Source: CAD feature listing. Evaluate the final solid. Frame: model axes, mm. A direction names the side the tool comes from. Coordinates: 2 decimals unless noted, no trailing zeros. Write each loop counter-clockwise with the first axis right and the second up, starting at its lowest first coordinate (ties: lowest second). Pieces come first, ordered by that corner, then holes. Notation, with made-up numbers: M 87.5,63.25 L 133.5,63.25 A28 cw 133.5,85.25 Z; hole C 10.5,-33 d5. An arc over 180 degrees is marked long. Answer as CSV lines item,"result". Start each with the question number.
1. Line query: probe 1 along Y at (x, z) = (-7.5, 484.05); probe 2 along Z at (x, y) = (-7.5, -4.25); probe 3 along Z at (x, y) = (7.5, -6.25). Output: solid intervals per line, ascending. Write a range as [from, to].
2. Contact query for flat-ended pins moving along their axis: pin 1 Ø1 at (x, z) = (0.5, 265.5) entering from +Y; pin 2 Ø1.5 at (x, z) = (-2, 96) entering from +Y; pin 3 Ø1.5 at (x, y) = (-4.5, -15) entering from +Z; pin 4 Ø0.6 at (x, z) = (1, 337.5) entering from -Y. Output: stop coordinate, or through.
3. Reachability of faces 4 (the face through (-7, -16, 0)), 5 (the face through (18.53, -8.73, 494.61)), 6 (the face through (16.5, -13.8, 480)) from +Z, -Z, +X, -X, +Y, -Y: full face, straight path, thin tool, end or side. Return the list, or none.
4. Mould query, pull axis Z, two halves, no side actions, for faces 1 (the face through (16, -15, 505)), 2 (the face through (0, -14, 243)), 3 (the face through (14, 0, 243)). Classes: pulls with the +Z half, pulls with the -Z half, needs draft (parallel to the pull), parting line crosses it, or undercut.
5. Section A-A on z = 353. Return the cut outline in (x, y), plus the area to 3 significant figures.
Autodesk Inventor part; units mm, degrees
ref_plane "YZ Plane" through (0, 0, 0) normal (1, 0, 0) x (0, 1, 0)
ref_plane "XZ Plane" through (0, 0, 0) normal (0, 1, 0) x (-1, 0, 0)
ref_plane "XY Plane" through (0, 0, 0) normal (0, 0, 1) x (1, 0, 0)
sketch "草图1" plane through (0, 0, 0) normal (0, 0, 1) x (1, 0, 0)
  arc A0 (0, -28) -> (28, 0) centre (0, 0) ccw
  line L0 (0, 0) -> (28, 0)
  line L1 (0, 0) -> (0, -28)
  dimension "d0" = 28
extrude "拉伸1" add sketch "草图1" along normal blind 480
shell "抽壳1" thickness 2 removed faces 1 at (13.1163, -13.1163, 480)
sketch "草图2" plane through (0, 0, 480) normal (0, 0, 1) x (1, 0, 0)
  line L0 (0, -28) -> (-15, -28)
  line L1 (-15, -28) -> (-15, 0)
  line L2 (-15, 0) -> (0, 0)
  line L3 (0, 0) -> (0, -28)
  line L4 (28, 0) -> (0, 0)
  arc A0 (0, -28) -> (28, 0) centre (0, 0) ccw
  line L5 (0, 0) -> (28, 0)
  line L6 (0, 0) -> (0, -28)
  line L7 (0, 0) -> (0, -28)
  dimension "d4" = 15
extrude "拉伸2" add sketch "草图2" along normal blind 5
sketch "草图3" plane through (0, 0, 485) normal (0, 0, 1) x (1, 0, 0)
  circle A0 centre (11.598, -11.598) radius 7.5
  circle A1 centre (11.598, -11.598) radius 11.598
  line L0 (28, 0) -> (-15, 0)
  line L1 (0, 0) -> (0, -28)
  arc A2 (0, -28) -> (28, 0) centre (0, 0) ccw
  dimension "d7" = 15
extrude "拉伸3" add sketch "草图3" along normal blind 20 contours A0
sketch "草图4" plane through (11.598, -11.598, 505) normal (0, 0, 1) x (1, 0, 0)
  circle A0 centre (0, 0) radius 5
  circle A1 centre (0, 0) radius 7.5
  point P0 (-11.598, 11.598)
  dimension "d10" = 10
extrude "拉伸4" cut sketch "草图4" against normal up to surface (25 mm away) contours A0
thread "螺纹1"
chamfer "倒角1" distance 0.5 angle 45 1 edges at (4.098, -11.598, 505)
sketch "草图5" plane through (0, 0, 0) normal (0, 0, -1) x (-1, 0, 0)
  arc A0 (-28, 0) -> (0, -28) centre (0, 0) ccw
  line L0 (-28, 0) -> (15, 0)
  line L1 (-28, 0) -> (15, 0)
  line L2 (15, 0) -> (15, -28)
  line L3 (15, 0) -> (15, -28)
  line L4 (15, -28) -> (0, -28)
  line L5 (15, -28) -> (0, -28)
  arc A1 (-25.923, -2) -> (-2, -25.923) centre (0, 0) ccw
extrude "拉伸5" add sketch "草图5" along normal blind 5
sketch "草图6" plane through (0, 0, 485) normal (0, 0, 1) x (1, 0, 0)
  circle A0 centre (-7.5, -9) radius 2.5
  circle A1 centre (-7.5, -23) radius 2.5
  line L0 (28, 0) -> (-15, 0)
  line L1 (-15, -28) -> (0, -28)
  line L2 (-15, 0) -> (-15, -28)
  point P0 (0, 0)
  dimension "d20" = 5
  dimension "d21" = 5
  dimension "d22" = 9
  dimension "d23" = 5
  dimension "d24" = 7.5
  dimension "d25" = 7.5
extrude "拉伸6" cut sketch "草图6" against normal through all
sketch "草图7" plane through (0, 0, 485) normal (0, 0, 1) x (1, 0, 0)
  line L0 (-15, 0) -> (0, 0)
  line L1 (0, 0) -> (0, -4)
  line L2 (0, -4) -> (-15, -4)
  line L3 (-15, -4) -> (-15, 0)
  line L4 (0, 0) -> (0, -28)
  line L5 (28, 0) -> (-15, 0)
  line L6 (-15, 0) -> (-15, -28)
  dimension "d28" = 4
extrude "拉伸7" cut sketch "草图7" against normal through all
sketch "草图8" plane through (0, 0, -5) normal (-1, 0, 0) x (0, 0, 1)
  line L0 (7, -25.923) -> (485, -25.923)
  line L1 (470, -25.923) -> (450, -25.923)
  line L2 (450, -25.923) -> (450, -23.923)
  line L3 (450, -23.923) -> (470, -23.923)
  line L4 (470, -23.923) -> (470, -25.923)
  line L5 (485, -4) -> (485, -28)
  point P0 (5, 0)
  dimension "d31" = 20
  dimension "d32" = 2
  dimension "d33" = 15
extrude "拉伸8" cut sketch "草图8" against normal blind 2
pattern_linear "矩形阵列1" count 2 spacing 70 along (0, 0, -1) of "拉伸8"
pattern_linear "矩形阵列2" count 4 spacing 120 along (0, 0, -1) of "拉伸8", "矩形阵列1"
properties part number "分离水箱"
Values:
1,probe 1,"[-28, -25.5], [-20.5, -11.5], [-6.5, -4]"
1,probe 2,"[-5, 0], [480, 485]"
1,probe 3,"[-5, 2], [480, 505]"
2,pin 1,"y = 0"
2,pin 2,"through"
2,pin 3,"z = 485"
2,pin 4,"y = -27.99"
3,face 4,"-X, +Y, -Y"
3,face 5,"+Z"
3,face 6,"none"
4,face 1,"pulls with the +Z half"
4,face 2,"undercut"
4,face 3,"needs draft"
5,outline,"M 0,-28 A28 ccw 28,0 L 0,0 Z; hole M 2,-25.92 A26 ccw 25.92,-2 L 2,-2 Z"
5,area,"185 mm²"
